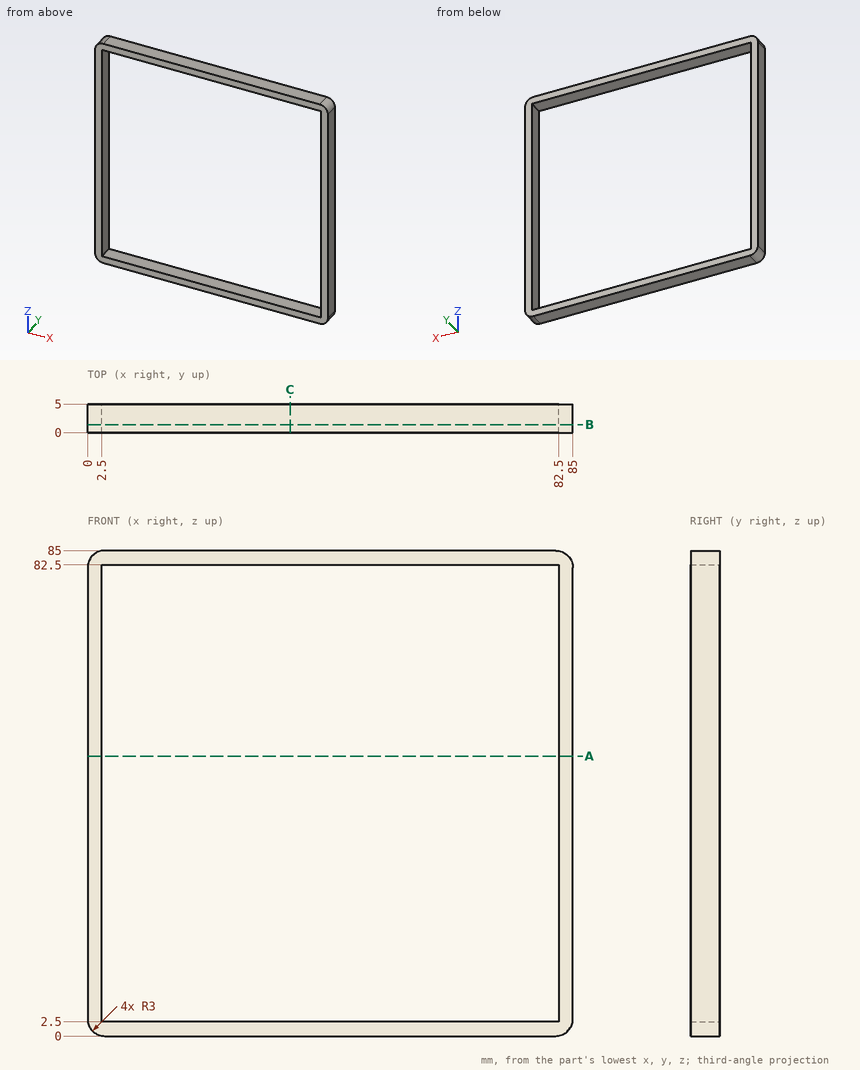
Check sheet for the drawn part. Datum: minimum x, y, z corner. Units: mm. Give positions to 0.01 mm unless a question says otherwise; leave off trailing zeros. Loops run counter-clockwise (first coordinate to the right, second up) from the corner with the lowest first, then second, coordinate; pieces in that order, holes last. Notation, with made-up numbers: (-27, 87) - (1, 87) arc R35 cw to (1, 123) - close; hole circle Ø1 at (81.5, 15). An arc over 180 degrees is marked (long way). Write each question's results on one line, items separated by ' | '.
1) Material ranges on L1, parallel to X at y = 1.3, z = 15, recorded low to high. Write a range as from..to.
Solution:
L1: 0..2.5, 82.5..85
2) Sectioned sample at A-A on z = 49. Record the boundary of the cut face in (x, y), plus the area to 3 significant figures.
Solution:
outline: (0, 0) - (2.5, 0) - (2.5, 5) - (0, 5) - close; (82.5, 0) - (85, 0) - (85, 5) - (82.5, 5) - close | area: 25.0 mm2
3) Sectioned sample at B-B on y = 1.4. Record the boundary of the cut face in (x, z).
Solution:
outline: (0, 3) arc R3 ccw to (3, 0) - (82, 0) arc R3 ccw to (85, 3) - (85, 82) arc R3 ccw to (82, 85) - (3, 85) arc R3 ccw to (0, 82) - close; hole (2.5, 2.5) - (82.5, 2.5) - (82.5, 82.5) - (2.5, 82.5) - close
4) Sectioned sample at C-C on x = 35.5. Record the boundary of the cut face in (y, z).
Solution:
outline: (0, 0) - (5, 0) - (5, 2.5) - (0, 2.5) - close; (0, 82.5) - (5, 82.5) - (5, 85) - (0, 85) - close
